Model file for the job. Use its own axes, mm. A direction names the side the tool comes from. Coordinates: 2 decimals unless noted, no trailing zeros. Order: outer loops, then holes, each group sorted by start corner. A loop starts at its lowest first (then second) coordinate and runs counter-clockwise, first axis right, second up.
from build123d import *

# Parameters (mm, degrees)
REVOLVE2_ANGLE                 = 180
CBORE_FOR_M2_SHCS1_D           = 2.2
CBORE_FOR_M2_SHCS1_CBORE_D     = 4.4
CBORE_FOR_M2_SHCS1_CBORE_DEPTH = 50
SKETCH13_R                     = 1.65
CUT_EXTRUDE2_DEPTH             = 100


with BuildPart() as part:
    # Sketch3 → Revolve2 (revolve)
    with BuildSketch(Plane.XY):
        Polygon((48.25, 0), (47.584421203, -12.7), (55, -12.7), (55, 0), align=None)
    revolve(axis=Axis((0, 50.355486862, 0), (0, -1, 0)), revolution_arc=REVOLVE2_ANGLE)

    # CBORE for M2 SHCS1 (through all)
    with Locations(Plane.XY.offset(55)):
        with Locations((51.625, -3.35), (51.625, -9.35)):
            cbore_for_m2_shcs1 = CounterBoreHole(CBORE_FOR_M2_SHCS1_D / 2, CBORE_FOR_M2_SHCS1_CBORE_D / 2, CBORE_FOR_M2_SHCS1_CBORE_DEPTH)

    # Mirror1: CBORE for M2 SHCS1 across plane
    add(cbore_for_m2_shcs1.mirror(Plane(origin=(0, 0, 0), x_dir=(0, 0, 1), z_dir=(1, 0, 0))), mode=Mode.SUBTRACT)

    # Sketch13 → Cut-Extrude2 (cut, symmetric)
    with BuildSketch(Plane(origin=(0, 0, 0), x_dir=(0.707106781, 0, 0.707106781), z_dir=(-0.707106781, 0, 0.707106781))):
        with Locations((0, -6.35)):
            Circle(SKETCH13_R)
    extrude(amount=CUT_EXTRUDE2_DEPTH, both=True, mode=Mode.SUBTRACT)


solid = part.part
Q1. Cut at C-C, the plane y = -3.35. List the corners of the cut face in (x, z) (3 decimals), plus the area to 3 significant figures.
Established:
outline: (-55, 0) - (-52.725, 0) - (-52.725, 5) - (-53.825, 5) - (-53.825, 11.308) arc R55 ccw to start; (-50.525, 0) - (-48.074, 0) arc R48.074 cw to (48.074, 0) - (50.525, 0) - (50.525, 5) - (49.425, 5) - (49.425, 24.128) arc R55 ccw to (-49.425, 24.128) - (-49.425, 5) - (-50.525, 5) - close; (52.725, 0) - (55, 0) arc R55 ccw to (53.825, 11.308) - (53.825, 5) - (52.725, 5) - close
area: 980 mm2
Q2. Which spindle directions (+Z, -Z, +X, -X, +Y, -Y) get a long thin tool onto all of the face, cutting with end or side? Do faces 4 (the face through (-49.427, -9.253, 12.575)), 5 (the face through (-37.56, -6.28, 35.23)). Say none if no direction does.
Established:
face 4: +Z
face 5: none
Q3. Cut at A-A, the plane y = -9.35. List the corners of the cut face in (x, z) (3 decimals).
Established:
outline: (-55, 0) - (-52.725, 0) - (-52.725, 5) - (-53.825, 5) - (-53.825, 11.308) arc R55 ccw to start; (-50.525, 0) - (-47.76, 0) arc R47.76 cw to (47.76, 0) - (50.525, 0) - (50.525, 5) - (49.425, 5) - (49.425, 24.128) arc R55 ccw to (-49.425, 24.128) - (-49.425, 5) - (-50.525, 5) - close; (52.725, 0) - (55, 0) arc R55 ccw to (53.825, 11.308) - (53.825, 5) - (52.725, 5) - close
Q4. Mould opens along Y. For faces 1 (the face through (-49.427, -3.253, 12.575)), 2 (the face through (1.052, -7.85, 47.827)), 3 (the face through (51, -6, 0)) say: pulls with the +Y half, pulls with the -Y half, needs draft (parallel to the pull), parting line crosses it, or undercut.
Established:
face 1: undercut
face 2: pulls with the +Y half
face 3: needs draft
Q5. Probe line 1 (X direction, y = -8.5, z = 11); line 2 (X direction, y = -8.25, z = 36); line 3 (X direction, y = -7, z = 27). List the from-to ranges inside material, lowest first.
Established:
line 1: x = -53.89 to -53.65, -49.6 to -46.52, 46.52 to 49.6, 53.65 to 53.89
line 2: x = -41.58 to -31.47, 31.47 to 41.58
line 3: x = -47.92 to -39.54, 39.54 to 47.92
Q6. Drop flat-ended pins along their axis: P1, Ø1.8, axis at x = -51.625, y = -9.35, coming from the +Z side; P2, Ø3, axis at x = -28.5, y = -10, coming from the -Z side; P3, Ø5.5, axis at x = -51.625, y = -3.35, coming from the +Z side; P4, Ø2.5, axis at x = 51.625, y = -9.35, coming from the +Z side. Give the stop position or say it passes through.
Established:
P1: passes through
P2: stops at z = 37.11
P3: stops at z = 25.22
P4: stops at z = 5
Q7. Cut at B-B, the plane z = 8.5. Count the separate pieces of the cut face and the enclosed holes in it, plus the area to 3 significant figures.
Established:
separate pieces: 2
enclosed holes: 4
area: 122 mm2
